```python
from build123d import *

# Parameters (mm, degrees)
F0_W     = 35.56
F0_H     = 35.56
F1_DEPTH = 6.35
F2_W     = 3.81
F2_H     = 2.54
F3_DEPTH = 3.81
F4_W     = 3.81
F4_H     = 2.54
F5_DEPTH = 3.81


with BuildPart() as f1:
    # F0 (on Front) → F1 (new body)
    with BuildSketch(Plane.XZ):
        Rectangle(F0_W, F0_H)
    extrude(amount=F1_DEPTH)

    # F2 (on face) → F3 (join)
    with BuildSketch(Plane.YZ.offset(17.78)):
        with Locations((-1.905, 10.16)):
            Rectangle(F2_W, F2_H)
        with Locations((-1.905, -10.16)):
            Rectangle(F2_W, F2_H)
    extrude(amount=F3_DEPTH)

    # F4 (on face) → F5 (join)
    with BuildSketch(Plane(origin=(-17.78, 0, 0), x_dir=(0, -1, 0), z_dir=(-1, 0, 0))):
        with Locations((1.905, 10.16)):
            Rectangle(F4_W, F4_H)
        with Locations((1.905, -10.16)):
            Rectangle(F4_W, F4_H)
    extrude(amount=F5_DEPTH)


solid = f1.part
```
Geometry check sheet. Reference: the model listing, model coordinates, mm. A direction names the side the tool comes from. Give positions to 0.01 mm unless a question says otherwise; leave off trailing zeros. Write each loop counter-clockwise with the first axis right and the second up, starting at its lowest first coordinate (ties: lowest second). Pieces come first, ordered by that corner, then holes.
1) Material ranges on L1, parallel to Z at x = 18, y = -0.5; L2, parallel to X at y = -1.5, z = 11.5, recorded low to high.
2) Section check C-C, the plane y = -3. Record the boundary of the cut face in (x, z), and give its area (3 significant figures).
3) Section check A-A, the plane x = -18.5. Record the boundary of the cut face in (y, z).
4) Section check D-D, the plane z = 2. Record the boundary of the cut face in (x, y).
5) Access from +Z, -Z, +X, -X, +Y, -Y to the whole of each face (thin tool, end or side, straight path). Record for faces 1 (the flat face through (-20, -2, -8.89)), 2 (the flat face through (20, -2, -8.89)), 3 (the flat face through (-20, -3.81, 10)), 4 (the flat face through (20, -2, 11.43)), 5 (the flat face through (20, -3.81, 10)).
6) Gauge pin test, flat ends, axial feed: pin 1 (1.9 mm diameter, centred on y = -3.5, z = -4.5, fed in from -X); pin 2 (12 mm diameter, centred on x = 2.5, z = -13, fed in from +Y); pin 3 (1.9 mm diameter, centred on x = 19, y = -2, fed in from +Z); pin 4 (1.3 mm diameter, centred on x = 20, z = -10, fed in from -Y). Record the tip position at first contact, or that the pin passes through.
7) Section check B-B, the plane z = -10. Record the boundary of the cut face in (x, y), and give its area (3 significant figures).
8) Release check for a two-part mould opening along Z. For faces 6 (the flat face through (21.59, -2, 10)), 7 (the flat face through (-20, -2, 11.43)), 8 (the flat face through (-20, -2, 8.89)) record: pulls with the +Z half, pulls with the -Z half, needs draft (parallel to the pull), parting line crosses it, or undercut.
Computed:
1. L1: z = -11.43 to -8.89, 8.89 to 11.43
1. L2: x = -17.78 to 17.78
2. outline: (-21.59, -11.43) - (-17.78, -11.43) - (-17.78, -17.78) - (17.78, -17.78) - (17.78, -11.43) - (21.59, -11.43) - (21.59, -8.89) - (17.78, -8.89) - (17.78, 8.89) - (21.59, 8.89) - (21.59, 11.43) - (17.78, 11.43) - (17.78, 17.78) - (-17.78, 17.78) - (-17.78, 11.43) - (-21.59, 11.43) - (-21.59, 8.89) - (-17.78, 8.89) - (-17.78, -8.89) - (-21.59, -8.89) - close
2. area: 1,300 mm2
3. outline: (-3.81, -11.43) - (0, -11.43) - (0, -8.89) - (-3.81, -8.89) - close; (-3.81, 8.89) - (0, 8.89) - (0, 11.43) - (-3.81, 11.43) - close
4. outline: (-17.78, -6.35) - (17.78, -6.35) - (17.78, 0) - (-17.78, 0) - close
5. face 1: -X, +Y, -Y
5. face 2: +X, +Y, -Y
5. face 3: +Z, -Z, -X, -Y
5. face 4: +Z, +X, +Y, -Y
5. face 5: +Z, -Z, +X, -Y
6. pin 1: stops at x = -17.78
6. pin 2: stops at y = 0
6. pin 3: stops at z = 11.43
6. pin 4: stops at y = -3.81
7. outline: (-21.59, -3.81) - (-17.78, -3.81) - (-17.78, -6.35) - (17.78, -6.35) - (17.78, -3.81) - (21.59, -3.81) - (21.59, 0) - (-21.59, 0) - close
7. area: 255 mm2
8. face 6: needs draft
8. face 7: pulls with the +Z half
8. face 8: undercut
